from build123d import *

# Parameters (mm, degrees)
F0_W        = 144
F0_H        = 120
F0_W_2      = 10
F0_H_2      = 110
F0_H_3      = 110.1521776617
F0_H_4      = 110.1521739364
F1_DEPTH    = 3.5
F2_R        = 2
F3_T1_DEPTH = 153.6824583655
F4_T1_DEPTH = 126.1270166538


# Not quite as in the source:
# - a fillet or chamfer that OpenCascade refuses, or shapes differently, is made with other operations: its cross-section is extruded or revolved along the edge and cut away or added


with BuildPart() as f1:
    # F0 (on Top) → F1 (new body)
    with BuildSketch(Plane.XY):
        Rectangle(F0_W, F0_H)
        with Locations((-63, 0)):
            Rectangle(F0_W_2, F0_H_2, mode=Mode.SUBTRACT)
        with Locations((-49, 0)):
            Rectangle(F0_W_2, F0_H_2, mode=Mode.SUBTRACT)
        with Locations((-35, 0.0760888308)):
            Rectangle(F0_W_2, F0_H_3, mode=Mode.SUBTRACT)
        with Locations((-21, 0.0760869682)):
            Rectangle(F0_W_2, F0_H_4, mode=Mode.SUBTRACT)
        with Locations((-7, 0.0760869682)):
            Rectangle(F0_W_2, F0_H_4, mode=Mode.SUBTRACT)
        with Locations((7, 0.0760869682)):
            Rectangle(F0_W_2, F0_H_4, mode=Mode.SUBTRACT)
        with Locations((21, 0.0760888308)):
            Rectangle(F0_W_2, F0_H_3, mode=Mode.SUBTRACT)
        with Locations((35, 0.0760869682)):
            Rectangle(F0_W_2, F0_H_4, mode=Mode.SUBTRACT)
        with Locations((49, 0.0760888308)):
            Rectangle(F0_W_2, F0_H_3, mode=Mode.SUBTRACT)
        with Locations((63, 0.0760888308)):
            Rectangle(F0_W_2, F0_H_3, mode=Mode.SUBTRACT)
    extrude(amount=F1_DEPTH)

    # F2
    f2_edges = [f1.edges().sort_by_distance(p)[0] for p in [
        (0, 60, 3.5),
        (0, -60, 3.5),
    ]]
    fillet(f2_edges, radius=F2_R)

    # F3: fillet of radius 2 on 2 edges, made by hand

    # F3_s2 → F3_t1 (cut)
    with BuildSketch(Plane.YZ.offset(-76.8412291828)):
        with BuildLine():
            ThreePointArc((-58.0635083269, 0), (-59.2882531983, 0.4188611699), (-60, 1.5))
            Line((-60, 1.5), (-60, 0))
            Line((-60, 0), (-58.0635083269, 0))
        make_face()
        with BuildLine():
            ThreePointArc((60, 1.5), (59.2882531983, 0.4188611699), (58.0635083269, 0))
            Line((58.0635083269, 0), (60, 0))
            Line((60, 0), (60, 1.5))
        make_face()
    extrude(amount=F3_T1_DEPTH, mode=Mode.SUBTRACT)

    # F4: fillet of radius 2 on 2 edges, made by hand

    # F4_s2 → F4_t1 (cut)
    with BuildSketch(Plane.XZ.offset(-63.0635083269)):
        with BuildLine():
            ThreePointArc((-72, 2), (-71.4142135624, 0.5857864376), (-70, 0))
            Line((-70, 0), (-72, 0))
            Line((-72, 0), (-72, 2))
        make_face()
        with BuildLine():
            ThreePointArc((72, 2), (71.4142135624, 0.5857864376), (70, 0))
            Line((70, 0), (72, 0))
            Line((72, 0), (72, 2))
        make_face()
    extrude(amount=F4_T1_DEPTH, mode=Mode.SUBTRACT)


solid = f1.part
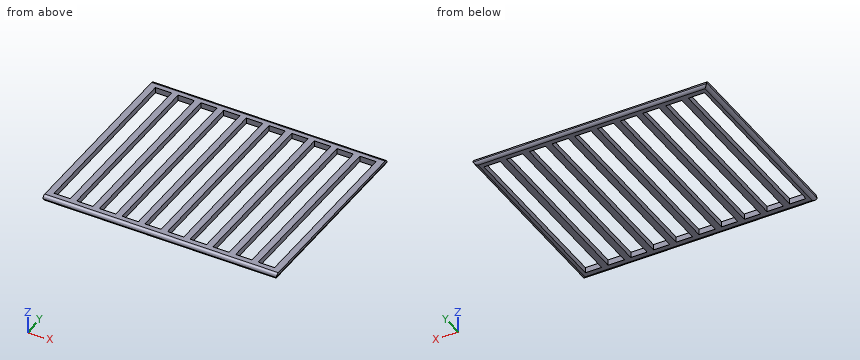
Source: CAD feature listing. Evaluate the final solid. Frame: model axes, mm. Coordinates: 2 decimals unless noted, no trailing zeros. Loops run counter-clockwise (first coordinate to the right, second up) from the corner with the lowest first, then second, coordinate; pieces in that order, holes last. Notation, with made-up numbers: (4, 38.5) -> (60, 38.5) arc R16 ccw to (60, 60.5) -> close; hole circle Ø1 at (54, 82.5). An arc over 180 degrees is marked (long way). Answer in a Markdown table with one row per item. Add a question column.
Q1. Section B-B on y = 49.5. Give the number of separate pieces and of enclosed holes in the cut face, and give its area (3 significant figures).
Q2. Ray query, line 1 along Y through (x, z) = (-3, 1.4); line 2 along Y through (x, z) = (-23, 1.3); line 3 along Y through (x, z) = (-40.5, 2.45). Return the intervals inside material, ascending.
Q3. Section A-A on x = -50. Return the cut outline in (y, z).
Q4. Contact query for flat-ended pins moving along their axis: pin 1 Ø1.5 at (y, z) = (-3, 1.5) entering from +X; pin 2 Ø1.8 at (x, z) = (-60.5, 2.5) entering from -Y. Output: stop coordinate, or through.
Q5. Section C-C on x = -8. Return the cut outline in (y, z), and give its area (3 significant figures).
Computed values:
| question | item | result |
|---|---|---|
| 1 | separate pieces | 11 |
| 1 | enclosed holes | 0 |
| 1 | area | 152 mm^2 |
| 2 | line 1 | y = -59.97 to -55, 55.15 to 59.97 |
| 2 | line 2 | y = -59.94 to -55, 55.15 to 59.94 |
| 2 | line 3 | y = -59.76 to 59.76 |
| 3 | outline | (-60, 1.5) arc R2 ccw to (-58.06, 0) -> (-55, 0) -> (-55, 3.5) -> (-58, 3.5) arc R2 ccw to start; (55, 0) -> (58.06, 0) arc R2 ccw to (60, 1.5) arc R2 ccw to (58, 3.5) -> (55, 3.5) -> close |
| 4 | pin 1 | stops at x = 72 |
| 4 | pin 2 | stops at y = -60 |
| 5 | outline | (-60, 1.5) arc R2 ccw to (-58.06, 0) -> (-55, 0) -> (-55, 3.5) -> (-58, 3.5) arc R2 ccw to start; (55.15, 0) -> (58.06, 0) arc R2 ccw to (60, 1.5) arc R2 ccw to (58, 3.5) -> (55.15, 3.5) -> close |
| 5 | area | 31.2 mm^2 |
